Autodesk Inventor part; units mm, degrees
ref_plane "YZ Plane" through (0, 0, 0) normal (1, 0, 0) x (0, 1, 0)
ref_plane "XZ Plane" through (0, 0, 0) normal (0, 1, 0) x (-1, 0, 0)
ref_plane "XY Plane" through (0, 0, 0) normal (0, 0, 1) x (1, 0, 0)
sketch "草图1" plane through (0, 0, 0) normal (0, 0, 1) x (1, 0, 0)
  circle A0 centre (0.6467, -2.2689) radius 2.75
  circle A1 centre (4.8161, 2.4002) radius 2.5 construction
  circle A2 centre (4.8161, 2.4002) radius 2.5 construction
  circle A3 centre (4.8161, 2.4002) radius 2.5 construction
  line L0 (16.9048, -7.8392) -> (-3.0952, -7.8392)
  line L1 (-3.0952, -7.8392) -> (-3.0952, -22.8392)
  line L2 (-3.0952, -22.8392) -> (16.9048, -22.8392)
  line L3 (16.9048, -22.8392) -> (16.9048, -7.8392)
  line L4 (16.9048, -6.8375) -> (16.9048, -82.9867)
  line L5 (-1.0952, -7.8392) -> (16.9048, -7.8392)
  line L6 (-3.0952, 9.1608) -> (11.9048, 9.1608)
  line L7 (11.9048, 9.1608) -> (11.9048, -22.8392)
  line L8 (11.9048, -22.8392) -> (-3.0952, -22.8392)
  line L9 (-3.0952, -22.8392) -> (-3.0952, 9.1608)
  circle A4 centre (4.8161, 2.4002) radius 2.75
  point P0 (-3.0952, -7.8392)
  point P1 (11.9048, -7.8392)
  dimension "d2" = 15
  dimension "d3" = 20
  dimension "d4" = 15
  dimension "d5" = 17
  dimension "d26" = 5.5
  dimension "d28" = 5.5
extrude "拉伸1" add sketch "草图1" against normal blind 12
move faces "移动1" translate (0, 0, -4) faces at (8.5714, -17.8392, 0)
sketch "草图3" plane through (-3.0952, -22.8392, -4) normal (0, 0, 1) x (1, 0, 0)
  line L0 (20, 15) -> (20, 0)
  line L1 (0, 0) -> (0, 32)
  line L2 (20, 0) -> (0, 0)
  line L3 (0, 0) -> (0, 15)
  line L4 (0, 15) -> (20, 15)
  line L5 (20, 15) -> (20, 0)
  line L6 (20, 15) -> (15, 15)
  point P0 (3.0952, 22.8392)
extrude "拉伸2" add sketch "草图3" along normal blind 10
chamfer "倒角1" distance 5 angle 45 1 edges at (11.9048, -7.8392, -8)
chamfer "倒角2" distance 1 angle 45 2 edges at (-3.0952, 9.1608, -8) (11.9048, 9.1608, -8)
sketch "草图4" plane through (16.9048, -22.8392, 6) normal (1, 0, 0) x (0, 0, -1)
  circle A0 centre (4, 7.5) radius 2
  line L0 (0, 15) -> (0, 0)
  line L1 (0, 7.5) -> (18, 7.5)
  line L2 (18, 0) -> (18, 31)
  circle A1 centre (14, 7.5) radius 2
  line L3 (0, 0) -> (0, 15)
  point P0 (6, 22.8392)
  point P1 (0, 7.5)
  dimension "d17" = 4
  dimension "d18" = 4
  dimension "d19" = 10
  dimension "d20" = 4
extrude "拉伸3" cut sketch "草图4" against normal blind 5
chamfer "倒角3" distance 2 angle 45 2 edges at (6.9048, -7.8392, 6) (6.9047, -7.8392, -4)
properties part number "滚纸"
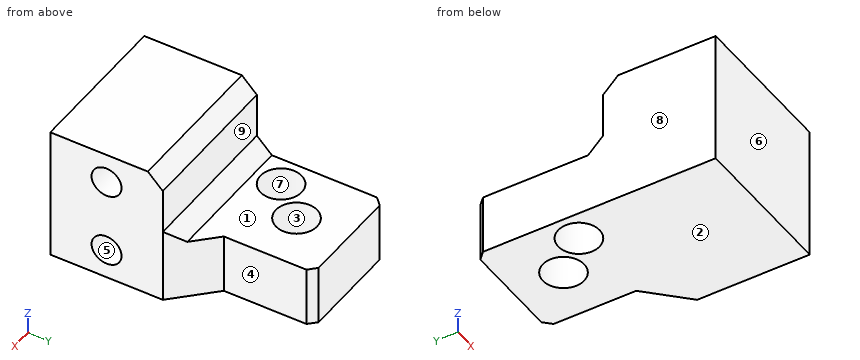
Work out the finished part from the listing and answer in its coordinate system (mm). Face numbers are marked on the shaded views. A direction names the side the tool comes from. Round coordinates to 2 decimals unless told otherwise and drop trailing zeros. Write each loop counter-clockwise with the first axis right and the second up, starting at its lowest first coordinate (ties: lowest second). Pieces come first, ordered by that corner, then holes. Notation, with made-up numbers: (73, -11) - (119, -11) arc R17 cw to (119, 0) - close; hole circle Ø8 at (-21.5, -35). An arc over 180 degrees is marked (long way). Answer in a Markdown table with one row per item. Add a question column.
1. For the marked faces 1, 2, 3, 4 and 5, determine the directions among +Z, -Z, +X, -X, +Y, -Y from which every point of the face is accessible in a straight line to the end or side of a thin tool.
2. Find the intervals of material crossed by line 1 along Z through (x, y) = (8, -1); line 2 along Y through (x, z) = (14.05, 2); line 3 along Y through (x, z) = (15.8, -8), in increasing order. Write a range as from..to.
3. A cutting plane is placed at D-D, the plane z = 2. Determine the outline of the cut face in (x, y), and give its area (3 significant figures).
4. A cutting plane is placed at A-A, the plane y = 1.5. Determine the outline of the cut face in (x, z).
5. A cutting plane is placed at C-C, the plane x = 0.5. Determine the outline of the cut face in (y, z).
6. Given pin 1 (2 mm diameter, centred on x = 12.5, z = -4.5, fed in from +Y); pin 2 (2 mm diameter, centred on y = -15, z = -8, fed in from +X); pin 3 (9 mm diameter, centred on x = 4.82, y = 2.4, fed in from -Z); pin 4 (1 mm diameter, centred on y = -6, z = -10, fed in from +X), each flat-ended and moving along its own axis, determine where each tip first touches the part or whether it passes through.
7. A cutting plane is placed at B-B, the plane z = -5.5. Count the separate pieces of the cut face and the enclosed holes in it, and give its area (3 significant figures).
8. The mould has two halves that part along Y. Classify the marked faces 6, 7, 8 and 9: +Y half, -Y half, draft (parallel to the pull), parting line (faces both ways), or undercut.
Worked out:
| question | item | result |
|---|---|---|
| 1 | face 1 | +Z, +X, -X, +Y |
| 1 | face 2 | -Z, +X, -X, +Y, -Y |
| 1 | face 3 | +Z, -Z |
| 1 | face 4 | +Z, -Z, +X, +Y |
| 1 | face 5 | +X |
| 2 | line 1 | -12..-4 |
| 2 | line 2 | -22.84..-17.34, -13.34..-7.84 |
| 2 | line 3 | -22.84..-17.34, -13.34..-6.73 |
| 3 | outline | (-3.1, -22.84) - (16.9, -22.84) - (16.9, -17.34) - (11.9, -17.34) - (11.9, -13.34) - (16.9, -13.34) - (16.9, -7.84) - (-3.1, -7.84) - close |
| 3 | area | 280 mm^2 |
| 4 | outline | (-3.1, -12) - (2.22, -12) - (2.22, -4) - (-3.1, -4) - close; (7.41, -12) - (11.9, -12) - (11.9, -4) - (7.41, -4) - close |
| 5 | outline | (-22.84, -12) - (-5.01, -12) - (-5.01, -4) - (-5.84, -4) - (-7.84, -2) - (-7.84, 4) - (-9.84, 6) - (-22.84, 6) - close; (0.48, -12) - (9.16, -12) - (9.16, -4) - (0.48, -4) - close |
| 6 | pin 1 | y = 8.57 |
| 6 | pin 2 | x = 11.9 |
| 6 | pin 3 | z = -12 |
| 6 | pin 4 | x = 15.57 |
| 7 | separate pieces | 1 |
| 7 | enclosed holes | 2 |
| 7 | area | 519 mm^2 |
| 8 | face 6 | -Y half |
| 8 | face 7 | undercut |
| 8 | face 8 | draft |
| 8 | face 9 | +Y half |
